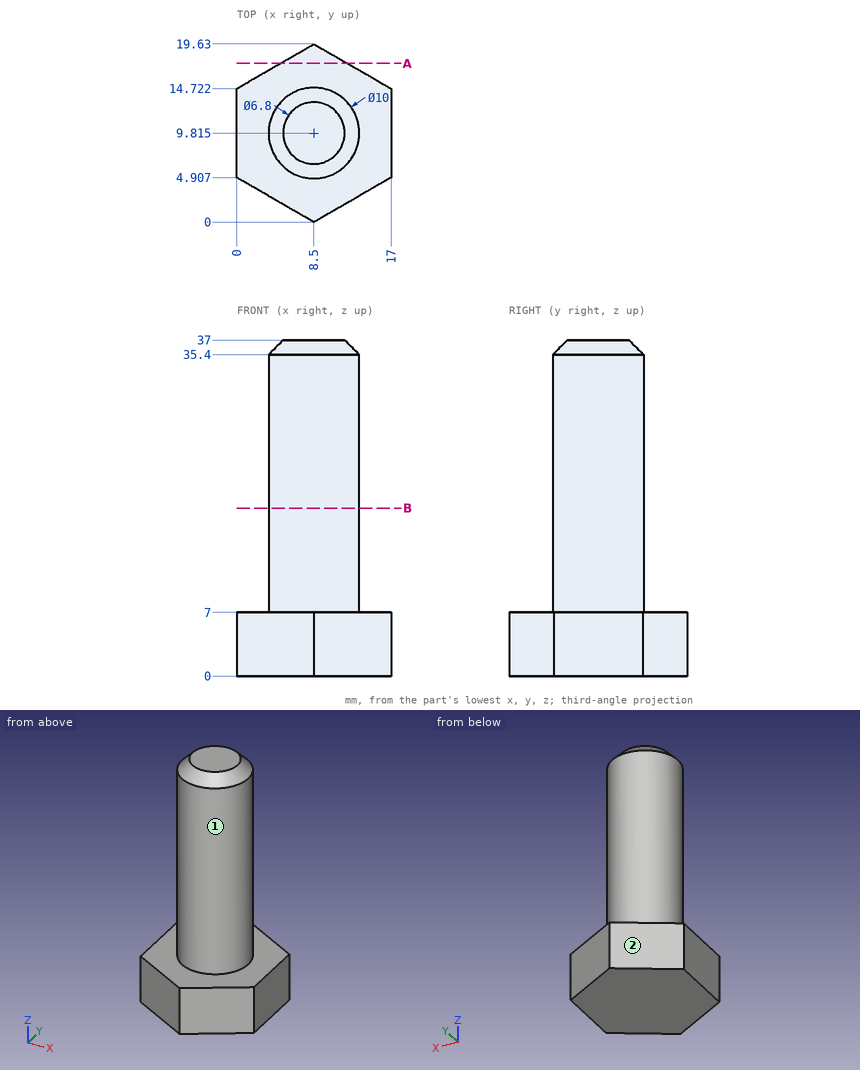
For this review, use the dimensioned drawing (mm, ordinates from the lowest corner) and the shaded views. A direction names the side the tool comes from. Coordinates: 2 decimals unless noted, no trailing zeros. Loops run counter-clockwise (first coordinate to the right, second up) from the corner with the lowest first, then second, coordinate; pieces in that order, holes last. Notation, with made-up numbers: (-4.5, 82) - (13.5, 82) arc R13 cw to (13.5, 93) - close; hole circle Ø7 at (-11.75, -37.75). An arc over 180 degrees is marked (long way). Use CSV: the item, a comma, the result in double quotes. Start each with the question number.
1) Consider section A-A on y = 17.5. Write out the cut boundary in (x, z).
2) Consider section B-B on z = 18.5. Write out the cut boundary in (x, y) (1 decimal).
3) Tool access review of the marked faces 1 and 2: name each direction out of +Z, -Z, +X, -X, +Y, -Y from which nothing blocks a thin tool from reaching the whole face with its end or side.
4) For pin 1 Ø1.5 at (x, z) = (7, 26.5) entering from +Y; pin 2 Ø1 at (x, z) = (10.5, 25) entering from +Y (1 decimal); pin 3 Ø10 at (x, z) = (14, 27.5) entering from -Y, all flat-tipped, find the tip position at first contact; note any pin that passes through.
5) Wall thickness on L1, parallel to Z at x = 14, y = 5.5; L2, parallel to X at y = 10, z = 25.5; L3, parallel to Y at x = 8.25, z = 15.5: over which ranges is each line inside the solid? List them lowest first. Write a range as from..to.
Geometry says:
1,outline,"(4.81, 0) - (12.19, 0) - (12.19, 7) - (4.81, 7) - close"
2,outline,"circle Ø10 at (8.5, 9.8)"
3,face 1,"+Z"
3,face 2,"+Z, -Z, -X, +Y"
4,pin 1,"y = 14.76"
4,pin 2,"y = 14.6"
4,pin 3,"y = 4.84"
5,L1,"0..7"
5,L2,"3.5..13.5"
5,L3,"4.82..14.81"
